Geometry check sheet. Reference: the model listing, model coordinates, mm. A direction names the side the tool comes from. Coordinates: 2 decimals unless noted, no trailing zeros. Order: outer loops, then holes, each group sorted by start corner. A loop starts at its lowest first (then second) coordinate and runs counter-clockwise, first axis right, second up. Notation, with made-up numbers: M 74,51.25 L 112,51.25 A19 ccw 112,81.25 Z; hole C 53.5,-2 d8. An arc over 180 degrees is marked long. Use CSV: the item, a comma, the result in double quotes. Start each with the question number.
```python
from build123d import *

# Parameters (mm, degrees)
F0_R     = 1.27
F1_DEPTH = 25.4
F3_DEPTH = 2.54
F5_DEPTH = 25.4


with BuildPart() as f1:
    # F0 (on Front) → F1 (new body)
    with BuildSketch(Plane.XZ):
        Circle(F0_R)
    extrude(amount=F1_DEPTH)

    # F2 (on face) → F3 (join)
    with BuildSketch(Plane.XZ.offset(25.4)):
        with BuildLine():
            ThreePointArc((-1.27, 0), (-0.898026, -0.898026), (0, -1.27))
            ThreePointArc((0, -1.27), (0.898026, -0.898026), (1.27, 0))
            ThreePointArc((1.27, 0), (0.898026, 0.898026), (0, 1.27))
            ThreePointArc((0, 1.27), (-0.898026, 0.898026), (-1.27, 0))
        make_face()
        with BuildLine():
            ThreePointArc((0, 1.27), (0.898026, 0.898026), (1.27, 0))
            Line((1.27, 0), (1.27, 1.27))
            Line((1.27, 1.27), (0, 1.27))
        make_face()
        with BuildLine():
            Line((0, -1.27), (1.27, -1.27))
            Line((1.27, -1.27), (1.27, 0))
            ThreePointArc((1.27, 0), (0.898026, -0.898026), (0, -1.27))
        make_face()
        with BuildLine():
            Line((-1.27, -1.27), (0, -1.27))
            ThreePointArc((0, -1.27), (-0.898026, -0.898026), (-1.27, 0))
            Line((-1.27, 0), (-1.27, -1.27))
        make_face()
        with BuildLine():
            Line((-1.27, 1.27), (-1.27, 0))
            ThreePointArc((-1.27, 0), (-0.898026, 0.898026), (0, 1.27))
            Line((0, 1.27), (-1.27, 1.27))
        make_face()
    extrude(amount=F3_DEPTH)

    # F4 (on face) → F5 (join)
    with BuildSketch(Plane.YZ.offset(1.27)):
        with BuildLine():
            Line((-27.94, 0), (-25.4, 0))
            ThreePointArc((-25.4, 0), (-25.771974, 0.898026), (-26.67, 1.27))
            ThreePointArc((-26.67, 1.27), (-27.568026, 0.898026), (-27.94, 0))
        make_face()
        with BuildLine():
            ThreePointArc((-26.67, -1.27), (-25.771974, -0.898026), (-25.4, 0))
            Line((-25.4, 0), (-27.94, 0))
            ThreePointArc((-27.94, 0), (-27.568026, -0.898026), (-26.67, -1.27))
        make_face()
    extrude(amount=F5_DEPTH)


solid = f1.part
```
1) Set-up check for faces 1 (the face through (-0.17, -12.52, 1.26)), 2 (the face through (-1.1, -25.4, 1)), 3 (the face through (1.27, -25.6, 1)), 4 (the face through (-1.01, -25.4, -1.01)): record each of +Z, -Z, +X, -X, +Y, -Y from which the full face is reachable in a straight line by a thin tool's end or side.
2) Material ranges on line 1 along Y through (x, z) = (7, -0.1); line 2 along X through (y, z) = (-10, -0.15); line 3 along X through (y, z) = (-9.25, -0.9), recorded low to high.
3) Section check A-A on z = 0.85. Record the boundary of the cut face in (x, y).
4) Section check D-D on z = -0.65. Record the boundary of the cut face in (x, y), then the cut area to 3 significant figures.
5) Gauge pin test, flat end, axial feed: P1, Ø5, axis at x = 23.5, y = -22.5, coming from the -Z side. Record the tip position at first contact, or that the pin passes through.
6) Section check B-B on x = 17.25. Record the boundary of the cut face in (y, z), then the cut area to 3 significant figures.
7) Section check C-C on y = -5.75. Record the boundary of the cut face in (x, z), then the cut area to 3 significant figures.
Results are:
1,face 1,"+Y"
1,face 2,"+Z, -X, +Y"
1,face 3,"+Z, +X, +Y"
1,face 4,"-Z, -X, +Y"
2,line 1,"y = -27.94 to -25.4"
2,line 2,"x = -1.26 to 1.26"
2,line 3,"x = -0.9 to 0.9"
3,outline,"M -1.27,-27.94 L 1.27,-27.94 L 1.27,-27.61 L 26.67,-27.61 L 26.67,-25.73 L 1.27,-25.73 L 1.27,-25.4 L 0.94,-25.4 L 0.94,0 L -0.94,0 L -0.94,-25.4 L -1.27,-25.4 Z"
4,outline,"M -1.27,-27.94 L 1.27,-27.94 L 1.27,-27.76 L 26.67,-27.76 L 26.67,-25.58 L 1.27,-25.58 L 1.27,-25.4 L 1.09,-25.4 L 1.09,0 L -1.09,0 L -1.09,-25.4 L -1.27,-25.4 Z"
4,area,"117 mm²"
5,P1,"passes through"
6,outline,"M -27.94,0 A1.27 ccw -26.67,-1.27 A1.27 ccw -25.4,0 A1.27 ccw -26.67,1.27 A1.27 ccw Z"
6,area,"5.07 mm²"
7,outline,"C 0,0 d2.54"
7,area,"5.07 mm²"
